from build123d import *

# Parameters (mm, degrees)
BASPROSKE_W         = 3
BASPROSKE_H         = 13.5
TOOTHCUT_DEPTH      = 20.32614809
TEETHCUTS_COUNT     = 25
HUBNEABOTSKE_R      = 3
HUBNEARBOTH_DEPTH   = 1.0000254
HUBFAR_START        = 1.0000254
HUBFARSKE_R         = 3
HUBFAR_DEPTH        = 1.0000254
BORSKE_R            = 1.5
BORE_DEPTH          = 5.0000508
BOSS_EXTRUDE1_START = 3
SKETCH1_R           = 3
SKETCH1_R_2         = 1.5
BOSS_EXTRUDE1_DEPTH = 3


with BuildPart() as part:
    # BasProSke → Base-Revolve (revolve)
    with BuildSketch(Plane(origin=(0, 0, 0), x_dir=(1, 0, 0), z_dir=(0, 1, 0)), mode=Mode.PRIVATE) as base_revolve_sk:
        with Locations((1.5, 6.75)):
            Rectangle(BASPROSKE_W, BASPROSKE_H)
    revolve(base_revolve_sk.sketch.rotate(Axis((-10, 0, 0), (1, 0, 0)), 180), axis=Axis((-10, 0, 0), (1, 0, 0)))

    # TooCutSke → ToothCut (cut, through all)
    with BuildSketch(Plane(origin=(0, 0, 0), x_dir=(0, 0, -1), z_dir=(1, 0, 0))):
        with BuildLine():
            ThreePointArc((0.570809389, 11.23450834), (0, 11.249), (-0.570809389, 11.23450834))
            ThreePointArc((-0.570809389, 11.23450834), (-0.823468719, 12.39261054), (-1.341642157, 13.4586939))
            ThreePointArc((-1.341642157, 13.4586939), (0, 13.5254), (1.341642157, 13.4586939))
            ThreePointArc((1.341642157, 13.4586939), (0.823468719, 12.39261054), (0.570809389, 11.23450834))
        make_face()
    toothcut = extrude(amount=TOOTHCUT_DEPTH, mode=Mode.SUBTRACT)

    # TeethCuts: ToothCut ×25 about axis
    teethcuts_axis = Axis((0, 0, 0), (1, 0, 0))
    for i in range(1, TEETHCUTS_COUNT):
        add(toothcut.rotate(teethcuts_axis, i * 360 / TEETHCUTS_COUNT), mode=Mode.SUBTRACT)

    # HubNeaBotSke → HubNearBoth (add)
    with BuildSketch(Plane.ZY):
        with Locations(Location((0, 0, 0), (0, 0, 180))):
            Circle(HUBNEABOTSKE_R)
    extrude(amount=HUBNEARBOTH_DEPTH)

    # HubFarSke → HubFar (add)
    with BuildSketch(Plane(origin=(3, 0, 0), x_dir=(0, 0, -1), z_dir=(1, 0, 0)).offset(HUBFAR_START)):
        Circle(HUBFARSKE_R)
    extrude(amount=-HUBFAR_DEPTH)

    # BorSke → Bore (cut, symmetric)
    with BuildSketch(Plane(origin=(0, 0, 0), x_dir=(0, 0, -1), z_dir=(1, 0, 0))):
        with Locations(Location((0, 0, 0), (0, 0, 180))):
            Circle(BORSKE_R)
    extrude(amount=BORE_DEPTH, both=True, mode=Mode.SUBTRACT)

    # Sketch1 → Boss-Extrude1 (add)
    with BuildSketch(Plane(origin=(4.0000254, 0, 0), x_dir=(0, 0, -1), z_dir=(1, 0, 0)).offset(BOSS_EXTRUDE1_START)):
        Circle(SKETCH1_R)
        with Locations(Location((0, 0, 0), (0, 0, 180))):
            Circle(SKETCH1_R_2, mode=Mode.SUBTRACT)
    extrude(amount=-BOSS_EXTRUDE1_DEPTH)


solid = part.part
Check sheet for the modelled part. Datum: model origin and axes. Units: mm. A direction names the side the tool comes from. Give positions to 0.01 mm unless a question says otherwise; leave off trailing zeros. Write each loop counter-clockwise with the first axis right and the second up, starting at its lowest first coordinate (ties: lowest second). Pieces come first, ordered by that corner, then holes. Notation, with made-up numbers: (25, 1.5) -> (51, 1.5) arc R27 cw to (51, 17.5) -> close; hole circle Ø6 at (46, 72). An arc over 180 degrees is marked (long way). One line per item, written item: value. Start each with the question number.
Item 1: Section check D-D on y = -8. Record the cut outline in (x, z).
Item 2: Material ranges on probe 1 along Z at (x, y) = (0.25, -11.75); probe 2 along Y at (x, z) = (3.5, 0); probe 3 along X at (y, z) = (6.75, 3.5), recorded low to high. Write a range as from..to.
Item 3: Section check A-A on z = 0. Record the cut outline in (x, y), then the cut area to 3 significant figures.
Item 4: Gauge pin test, flat ends, axial feed: pin 1 (10 mm diameter, centred on y = -2.5, z = -10.5, fed in from +X); pin 2 (12 mm diameter, centred on y = 4, z = 6, fed in from -X); pin 3 (8 mm diameter, centred on y = 9.5, z = -4.5, fed in from -X). Record the tip position at first contact, or that the pin passes through.
Item 5: Tool access check on faces 1 (the cylindrical face through (1.48, 9.57, -7.87)), 2 (the cylindrical face through (1.48, -11.16, -1.4)), 3 (the cylindrical face through (1.479, 10.442, 6.669)). Record the directions out of +Z, -Z, +X, -X, +Y, -Y that give a thin tool (end or side, any length) a straight path to the whole face; none if there is none.
Item 6: Section check B-B on x = 5. Record the cut outline in (y, z), then the cut area to 3 significant figures.
Item 7: Section check C-C on y = -2.25. Record the cut outline in (x, z), then the cut area to 3 significant figures.
Results list:
1. outline: (0, -8.65) -> (3, -8.65) -> (3, 8.65) -> (0, 8.65) -> close
2. probe 1: -6.65..-5.86, -3.79..-2.18, -0.83..0.83, 2.18..3.79, 5.86..6.65
2. probe 2: -3..-1.5, 1.5..3
2. probe 3: 0..3
3. outline: (-1, -3) -> (0, -3) -> (0, -13.5) -> (3, -13.5) -> (3, -3) -> (7, -3) -> (7, -1.5) -> (-1, -1.5) -> close; (-1, 1.5) -> (7, 1.5) -> (7, 3) -> (3, 3) -> (3, 11.25) -> (0, 11.25) -> (0, 3) -> (-1, 3) -> close
3. area: 80.2 mm²
4. pin 1: x = 3
4. pin 2: x = -1
4. pin 3: x = 0
5. face 1: +X, -X
5. face 2: +X, -X, -Y
5. face 3: +X, -X, +Y
6. outline: circle Ø6 at (0, 0); hole circle Ø3 at (0, 0)
6. area: 21.2 mm²
7. outline: (-1, -1.98) -> (0, -1.98) -> (0, -11.02) -> (3, -11.02) -> (3, -1.98) -> (7, -1.98) -> (7, 1.98) -> (3, 1.98) -> (3, 11.02) -> (0, 11.02) -> (0, 1.98) -> (-1, 1.98) -> close
7. area: 86.0 mm²
